The listing builds one solid part. Answer for the finished solid, in the listing's coordinates (mm). Face numbers are marked on the shaded views. A direction names the side the tool comes from. Give positions to 0.01 mm unless a question says otherwise; leave off trailing zeros. Write each loop counter-clockwise with the first axis right and the second up, starting at its lowest first coordinate (ties: lowest second). Pieces come first, ordered by that corner, then holes. Notation, with made-up numbers: M 3.25,-40 L 61.25,-40 A13 ccw 61.25,-32 Z; hole C 52,-21.75 d5. An arc over 180 degrees is marked long. Answer as a JSON object with one key per item and string values.
```python
from build123d import *

# Parameters (mm, degrees)
ESBO_O1_W                = 30
ESBO_O1_H                = 30
ESBO_O1_R                = 1.5
RESSALTO_EXTRUS_O1_DEPTH = 4
CORTE_EXTRUS_O1_REACH    = 23.587
ESBO_O2_R                = 9
ESBO_O4_R                = 12.95
CORTE_EXTRUS_O2_DEPTH    = 2


with BuildPart() as part:
    # Esboço1 → Ressalto-extrusão1 (new body)
    with BuildSketch(Plane.XY):
        Rectangle(ESBO_O1_W, ESBO_O1_H)
        with Locations((-12, -12)):
            Circle(ESBO_O1_R, mode=Mode.SUBTRACT)
        with Locations(Location((12, -12, 0), (0, 0, 180))):
            Circle(ESBO_O1_R, mode=Mode.SUBTRACT)
        with Locations((12, 12)):
            Circle(ESBO_O1_R, mode=Mode.SUBTRACT)
        with Locations(Location((-12, 12, 0), (0, 0, 180))):
            Circle(ESBO_O1_R, mode=Mode.SUBTRACT)
    extrude(amount=RESSALTO_EXTRUS_O1_DEPTH)

    # Esboço2 → Corte-extrusão1 (cut, up to next)
    with BuildSketch(Plane.XY.offset(4), mode=Mode.PRIVATE) as corte_extrus_o1_sk1:
        Circle(ESBO_O2_R)
    corte_extrus_o1_tool1 = extrude(corte_extrus_o1_sk1.sketch, amount=-CORTE_EXTRUS_O1_REACH, mode=Mode.PRIVATE) & part.part
    add(corte_extrus_o1_tool1.solids().sort_by_distance((0, 0, 4))[0], mode=Mode.SUBTRACT)

    # Esboço4 → Corte-extrusão2 (cut)
    with BuildSketch(Plane.XY.offset(4)):
        Circle(ESBO_O4_R)
    extrude(amount=-CORTE_EXTRUS_O2_DEPTH, mode=Mode.SUBTRACT)


solid = part.part
```
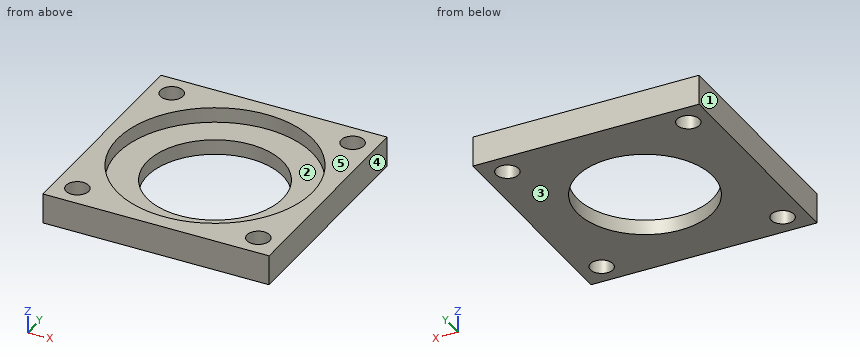
1. A cutting plane is placed at D-D, the plane y = 12. Give the vertices of the cut face in (x, z).
Verdict:
{"outline": "M -15,0 L -13.5,0 L -13.5,4 L -15,4 Z; M -10.5,0 L 10.5,0 L 10.5,4 L 4.87,4 L 4.87,2 L -4.87,2 L -4.87,4 L -10.5,4 Z; M 13.5,0 L 15,0 L 15,4 L 13.5,4 Z"}
2. A cutting plane is placed at A-A, the plane y = 0. Give the vertices of the cut face in (x, z), plus the area to 3 significant figures.
Verdict:
{"outline": "M -15,0 L -9,0 L -9,2 L -12.95,2 L -12.95,4 L -15,4 Z; M 9,0 L 15,0 L 15,4 L 12.95,4 L 12.95,2 L 9,2 Z", "area": "32.2 mm2"}
3. A cutting plane is placed at B-B, the plane z = 2.5. Give the vertices of the cut face in (x, y), plus the area to 3 significant figures.
Verdict:
{"outline": "M -15,-15 L 15,-15 L 15,15 L -15,15 Z; hole C -12,-12 d3; hole C -12,12 d3; hole C 0,0 d25.9; hole C 12,-12 d3; hole C 12,12 d3", "area": "345 mm2"}
4. A flat-ended cylindrical pin translates along its axis: pin 1 (1 mm diameter, centred on x = -6, y = 7, fed in from +Z). Find the tip coordinate at first contact, or state that the pin passes through.
Verdict:
{"pin 1": "stops at z = 2"}
5. The mould has two halves that part along Z. Classify the marked faces 3, 4 and 5: released by +Z, released by -Z, zero draft, split by the parting line, or undercut.
Verdict:
{"face 3": "released by -Z", "face 4": "zero draft", "face 5": "released by +Z"}
6. A cutting plane is placed at C-C, the plane x = -6.75. Give the vertices of the cut face in (y, z), plus the area to 3 significant figures.
Verdict:
{"outline": "M -15,0 L -5.95,0 L -5.95,2 L -11.05,2 L -11.05,4 L -15,4 Z; M 5.95,0 L 15,0 L 15,4 L 11.05,4 L 11.05,2 L 5.95,2 Z", "area": "52.0 mm2"}
7. Consider line 1 along Y through (x, z) = (12, 1.5); line 2 along Y through (x, z) = (-11.5, 0.35); line 3 along Y through (x, z) = (0, 3.1). Determine where each line is inside the solid, lowest interval first.
Verdict:
{"line 1": "y = -15 to -13.5, -10.5 to 10.5, 13.5 to 15", "line 2": "y = -15 to -13.41, -10.59 to 10.59, 13.41 to 15", "line 3": "y = -15 to -12.95, 12.95 to 15"}
8. For the marked faces 1 and 2, determine the directions among +Z, -Z, +X, -X, +Y, -Y from which every point of the face is accessible in a straight line to the end or side of a thin tool.
Verdict:
{"face 1": "+Z, -Z, -X, +Y, -Y", "face 2": "+Z"}
